For this review, take the finished solid that the model builds, in its own axes (mm). Face numbers are marked on the shaded views. Round coordinates to 2 decimals unless told otherwise and drop trailing zeros. Write each loop counter-clockwise with the first axis right and the second up, starting at its lowest first coordinate (ties: lowest second). Pieces come first, ordered by that corner, then holes.
from build123d import *

# Parameters (mm, degrees)
SKETCH1_W           = 800
SKETCH1_H           = 583
BOSS_EXTRUDE1_DEPTH = 1798.93
SKETCH2_R           = 16
BOSS_EXTRUDE2_DEPTH = 260
LPATTERN1_COUNT     = 2
LPATTERN1_PITCH     = 250
BOSS_EXTRUDE4_DEPTH = 30
LPATTERN3_COUNT     = 2
LPATTERN3_PITCH     = 1768.93
FILLET1_R           = 2


with BuildPart() as part:
    # Sketch1 → Boss-Extrude1 (new body)
    with BuildSketch(Plane(origin=(0, 0, 0), x_dir=(0, 0, -1), z_dir=(1, 0, 0))):
        with Locations((400, 291.5)):
            Rectangle(SKETCH1_W, SKETCH1_H)
    extrude(amount=BOSS_EXTRUDE1_DEPTH)

    # Sketch2 → Boss-Extrude2 (add)
    with BuildSketch(Plane(origin=(0, 583, 0), x_dir=(1, 0, 0), z_dir=(0, 1, 0))):
        with Locations(Location((1572.09, 179.8, 0), (0, 0, 90))):
            Circle(SKETCH2_R)
    boss_extrude2 = extrude(amount=BOSS_EXTRUDE2_DEPTH)

    # LPattern1: Boss-Extrude2 ×2
    with Locations(*[(-i * LPATTERN1_PITCH, 0, 0) for i in range(1, LPATTERN1_COUNT)]):
        add(boss_extrude2)

    # Sketch3 → Boss-Extrude4 (add)
    with BuildSketch(Plane.ZY):
        with BuildLine():
            Line((0, 174.272998957), (5, 174.272998957))
            ThreePointArc((5, 174.272998957), (26.213203436, 183.059795522), (35, 204.272998957))
            Line((35, 204.272998957), (35, 654.272998957))
            ThreePointArc((35, 654.272998957), (40.857864376, 668.415134581), (55, 674.272998957))
            Line((55, 674.272998957), (65, 674.272998957))
            ThreePointArc((65, 674.272998957), (79.142135624, 668.415134581), (85, 654.272998957))
            Line((85, 654.272998957), (85, 204.272998957))
            ThreePointArc((85, 204.272998957), (93.786796564, 183.059795522), (115, 174.272998957))
            Line((115, 174.272998957), (313.77, 174.272998957))
            ThreePointArc((313.77, 174.272998957), (334.983203436, 183.059795522), (343.77, 204.272998957))
            Line((343.77, 204.272998957), (343.77, 654.272998957))
            ThreePointArc((343.77, 654.272998957), (349.627864376, 668.415134581), (363.77, 674.272998957))
            Line((363.77, 674.272998957), (373.77, 674.272998957))
            ThreePointArc((373.77, 674.272998957), (387.912135624, 668.415134581), (393.77, 654.272998957))
            Line((393.77, 654.272998957), (393.77, 154.272998957))
            ThreePointArc((393.77, 154.272998957), (384.983203436, 133.059795522), (363.77, 124.272998957))
            Line((363.77, 124.272998957), (0, 124.272998957))
            Line((0, 124.272998957), (0, 174.272998957))
        make_face()
    boss_extrude4 = extrude(amount=-BOSS_EXTRUDE4_DEPTH)

    # LPattern3: Boss-Extrude4 ×2
    with Locations(*[(i * LPATTERN3_PITCH, 0, 0) for i in range(1, LPATTERN3_COUNT)]):
        add(boss_extrude4)

    # Fillet1
    fillet1_edges = [part.edges().sort_by_distance(p)[0] for p in [
        (1572.09, 843, -163.8),
        (1322.09, 843, -163.8),
    ]]
    fillet(fillet1_edges, radius=FILLET1_R)


solid = part.part
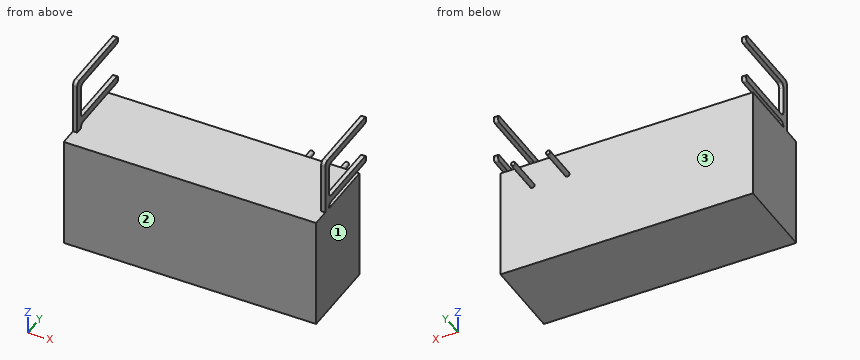
(1) Mouldability with a two-part tool opening along Y and no side actions: class the marked faces 1, 2 and 3 as pulls with the +Y half, pulls with the -Y half, needs draft (parallel to the pull), parting line crosses it, or undercut.
Geometry check:
face 1: needs draft
face 2: pulls with the -Y half
face 3: pulls with the +Y half
(2) We need section B-B, the plane y = 534.5. Give the boundary of the cut face in (x, z).
Geometry check:
outline: (0, -800) - (1798.93, -800) - (1798.93, 0) - (0, 0) - close; (0, 35) - (30, 35) - (30, 85) - (0, 85) - close; (0, 343.77) - (30, 343.77) - (30, 393.77) - (0, 393.77) - close; (1768.93, 35) - (1798.93, 35) - (1798.93, 85) - (1768.93, 85) - close; (1768.93, 343.77) - (1798.93, 343.77) - (1798.93, 393.77) - (1768.93, 393.77) - close
(3) We need section D-D, the plane z = -660.5. Give the boundary of the cut face in (x, y).
Geometry check:
outline: (0, 0) - (1798.93, 0) - (1798.93, 583) - (0, 583) - close
(4) We need section C-C, the plane y = 783. Give the boundary of the cut face in (x, z), and give its area (3 significant figures).
Geometry check:
outline: circle Ø32 at (1322.09, -179.8); circle Ø32 at (1572.09, -179.8)
area: 1,610 mm2
(5) For line 1 along Y through (x, z) = (178, -699.5); line 2 along Z through (x, y) = (594, 216), list the stretches that pass through material, from the lowest coordinate up.
Geometry check:
line 1: y = 0 to 583
line 2: z = -800 to 0
(6) We need section A-A, the plane z = 191. Give the boundary of the cut face in (x, y).
Geometry check:
outline: (0, 124.27) - (30, 124.27) - (30, 174.27) - (0, 174.27) - close; (1768.93, 124.27) - (1798.93, 124.27) - (1798.93, 174.27) - (1768.93, 174.27) - close
(7) For pin 1 Ø15 at (x, z) = (22, 229.5) entering from -Y; pin 2 Ø9 at (x, z) = (22, 182.5) entering from +Y; pin 3 Ø10 at (x, y) = (278, 557.5) entering from +Z, all flat-tipped, find the tip position at first contact; note any pin that passes through.
Geometry check:
pin 1: stops at y = 124.27
pin 2: stops at y = 174.27
pin 3: stops at z = 0
